```python
from build123d import *

# Parameters (mm, degrees)
BASE_FLANGE1_DEPTH = 44.45
CUT_EXTRUDE3_REACH = 107.213
SKETCH5_R          = 3.175


# Sheet-metal steps are written as plain solids
with BuildPart() as part:
    # Sketch1 → Base-Flange1 (new body)
    with BuildSketch(Plane.XY):
        with BuildLine():
            Line((-2.3368, 95.25), (-2.3368, 89.163964543))
            ThreePointArc((-2.3368, 89.163964543), (-1.962474978, 87.766964543), (-0.9398, 86.744289565))
            Line((-0.9398, 86.744289565), (-0.254, 86.34834275))
            ThreePointArc((-0.254, 86.34834275), (-0.068059095, 86.162401845), (0, 85.908401845))
            Line((0, 85.908401845), (0, -85.908401845))
            ThreePointArc((0, -85.908401845), (-0.068059095, -86.162401845), (-0.254, -86.34834275))
            Line((-0.254, -86.34834275), (-0.9398, -86.744289565))
            ThreePointArc((-0.9398, -86.744289565), (-1.962474978, -87.766964543), (-2.3368, -89.163964543))
            Line((-2.3368, -89.163964543), (-2.3368, -95.25))
            Line((-2.3368, -95.25), (-0.0508, -95.25))
            Line((-0.0508, -95.25), (-0.0508, -89.163964543))
            ThreePointArc((-0.0508, -89.163964543), (0.017259095, -88.909964543), (0.2032, -88.724023638))
            Line((0.2032, -88.724023638), (0.889, -88.328076823))
            ThreePointArc((0.889, -88.328076823), (1.911674978, -87.305401845), (2.286, -85.908401845))
            Line((2.286, -85.908401845), (2.286, 85.908401845))
            ThreePointArc((2.286, 85.908401845), (1.911674978, 87.305401845), (0.889, 88.328076823))
            Line((0.889, 88.328076823), (0.2032, 88.724023638))
            ThreePointArc((0.2032, 88.724023638), (0.017259095, 88.909964543), (-0.0508, 89.163964543))
            Line((-0.0508, 89.163964543), (-0.0508, 95.25))
            Line((-0.0508, 95.25), (-2.3368, 95.25))
        make_face()
    extrude(amount=BASE_FLANGE1_DEPTH)

    # Sketch5 → Cut-Extrude3 (cut, up to next)
    with BuildSketch(Plane(origin=(2.286, 0, 0), x_dir=(0, 0, -1), z_dir=(1, 0, 0)), mode=Mode.PRIVATE) as cut_extrude3_sk1:
        with Locations(Location((-22.225, 0, 0), (0, 0, 90))):
            Circle(SKETCH5_R)
    cut_extrude3_tool1 = extrude(cut_extrude3_sk1.sketch, amount=-CUT_EXTRUDE3_REACH, mode=Mode.PRIVATE) & part.part
    add(cut_extrude3_tool1.solids().sort_by_distance((2.286, 0, 22.225))[0], mode=Mode.SUBTRACT)


solid = part.part
```
Geometry: final body of the model. Coordinates: model frame, mm. A direction names the side the tool comes from. Give positions to 0.01 mm unless a question says otherwise; leave off trailing zeros. Write each loop counter-clockwise with the first axis right and the second up, starting at its lowest first coordinate (ties: lowest second). Pieces come first, ordered by that corner, then holes.
1. Pin query (flat end, axial travel): P1, Ø3, axis at y = 92.5, z = 29, coming from the +X side; P2, Ø1.5, axis at y = 47.5, z = 34.5, coming from the -X side. Return the tip coordinate at first contact, or that it passes through.
2. Line query: probe 1 along Z at (x, y) = (1.4, 0); probe 2 along Y at (x, z) = (-1, 42); probe 3 along Y at (x, z) = (-0.9, 12.5). Output: solid intervals per line, ascending.
3. Section query B-B, the plane z = 13.5. Return loops of the section in (x, y), then the cut area to 3 significant figures.
4. Section query A-A, the plane y = 0. Return loops of the section in (x, z).
5. Reachability of faces 1 (the flat face through (0, 1, 17)), 2 (the flat face through (-0.051, 92, 22)), 3 (the flat face through (-2.337, 92, 22)) from +Z, -Z, +X, -X, +Y, -Y: full face, straight path, thin tool, end or side. Return the list, or none.
6. Draft query along Z for faces 4 (the flat face through (1, 1, 0)), 5 (the cylindrical face through (1.159, -0.413, 25.373)), 6 (the flat face through (1, 1, 44.45)), 7 (the flat face through (-0.051, -92, 22)). Return one class per face: released by +Z, released by -Z, zero draft, split by the parting line, or undercut.
Computed:
1. P1: stops at x = -0.05
1. P2: stops at x = 0
2. probe 1: z = 0 to 19.05, 25.4 to 44.45
2. probe 2: y = -95.25 to -86.78, 86.78 to 95.25
2. probe 3: y = -95.25 to -86.72, 86.72 to 95.25
3. outline: (-2.34, -95.25) - (-0.05, -95.25) - (-0.05, -89.16) arc R0.51 cw to (0.2, -88.72) - (0.89, -88.33) arc R2.79 ccw to (2.29, -85.91) - (2.29, 85.91) arc R2.79 ccw to (0.89, 88.33) - (0.2, 88.72) arc R0.51 cw to (-0.05, 89.16) - (-0.05, 95.25) - (-2.34, 95.25) - (-2.34, 89.16) arc R2.79 ccw to (-0.94, 86.74) - (-0.25, 86.35) arc R0.51 cw to (0, 85.91) - (0, -85.91) arc R0.51 cw to (-0.25, -86.35) - (-0.94, -86.74) arc R2.79 ccw to (-2.34, -89.16) - close
3. area: 440 mm2
4. outline: (0, 0) - (2.29, 0) - (2.29, 19.05) - (0, 19.05) - close; (0, 25.4) - (2.29, 25.4) - (2.29, 44.45) - (0, 44.45) - close
5. face 1: +Z, -Z, -X
5. face 2: +Z, -Z, +X, +Y
5. face 3: +Z, -Z, -X, +Y, -Y
6. face 4: released by -Z
6. face 5: undercut
6. face 6: released by +Z
6. face 7: zero draft
